Input: part model. Units: mm. Frame: model coordinates. Face numbers are marked on the shaded views. Give positions to 0.01 mm unless a question says otherwise; leave off trailing zeros. Loops run counter-clockwise (first coordinate to the right, second up) from the corner with the lowest first, then second, coordinate; pieces in that order, holes last. Notation, with made-up numbers: (66.25, 69.25) -> (97.25, 69.25) arc R26 cw to (97.25, 89.25) -> close; hole circle Ø8 at (-22.75, 75). An arc over 180 degrees is marked (long way). One line per question, with ' | ' between items.
from build123d import *

# Parameters (mm, degrees)
BOSS_EXTRUDE1_START     = -10.5
SKETCH2_R               = 3.9
BOSS_EXTRUDE1_DEPTH     = 4
BOSS_EXTRUDE2_START     = -15.5
BOSS_EXTRUDE2_OUTLINE_R = 3.9
BOSS_EXTRUDE2_DEPTH     = 5
M3_CLEARANCE_HOLE1_D    = 3.2
M3_TAPPED_HOLE1_REACH   = 32.031
M3_TAPPED_HOLE1_BORE_R  = 1.25


# Read off the part's stored shape, not the designer's step: Boss-Extrude2
with BuildPart() as part:
    # Sketch2 → Boss-Extrude1 (new body)
    with BuildSketch(Plane(origin=(0, 0, 0), x_dir=(0, 0, -1), z_dir=(1, 0, 0)).offset(BOSS_EXTRUDE1_START)):
        with BuildLine():
            Line((7.534547605, -3.521676906), (13.278030312, -2.987088741))
            ThreePointArc((13.278030312, -2.987088741), (15.983180385, -0.317229866), (13.9, 2.861817604))
            Line((13.9, 2.861817604), (3.358528015, 6.176957176))
            Line((3.358528015, 6.176957176), (-4.343824749, 12.551142838))
            ThreePointArc((-4.343824749, 12.551142838), (-7.820620852, 12.799917558), (-9.185849324, 9.592714537))
            Line((-9.185849324, 9.592714537), (-6.737511079, -1.488604871))
            ThreePointArc((-6.737511079, -1.488604871), (-6.093212803, -3.237708717), (-5.004243793, -4.750530924))
            ThreePointArc((-5.004243793, -4.750530924), (-4.613436828, -5.232032538), (-4.301751563, -5.768153965))
            ThreePointArc((-4.301751563, -5.768153965), (-3.563882529, -6.593562507), (-2.5, -6.9))
            Line((-2.5, -6.9), (2.5, -6.9))
            ThreePointArc((2.5, -6.9), (3.563882529, -6.593562507), (4.301751563, -5.768153965))
            ThreePointArc((4.301751563, -5.768153965), (5.622657157, -4.219686633), (7.534547605, -3.521676906))
        make_face()
        Circle(SKETCH2_R, mode=Mode.SUBTRACT)
    extrude(amount=BOSS_EXTRUDE1_DEPTH)

    # Boss-Extrude2 outline → Boss-Extrude2 (add)
    with BuildSketch(Plane(origin=(0, 0, 0), x_dir=(0, 0, -1), z_dir=(1, 0, 0)).offset(BOSS_EXTRUDE2_START)):
        with BuildLine():
            ThreePointArc((5.004243793, -4.750530924), (0, 6.9), (-5.004243793, -4.750530924))
            ThreePointArc((-5.004243793, -4.750530924), (-4.613436828, -5.232032538), (-4.301751563, -5.768153965))
            ThreePointArc((-4.301751563, -5.768153965), (-3.563882529, -6.593562507), (-2.5, -6.9))
            Line((-2.5, -6.9), (2.5, -6.9))
            ThreePointArc((2.5, -6.9), (3.563882529, -6.593562507), (4.301751563, -5.768153965))
            ThreePointArc((4.301751563, -5.768153965), (4.613436828, -5.232032538), (5.004243793, -4.750530924))
        make_face()
        Circle(BOSS_EXTRUDE2_OUTLINE_R, mode=Mode.SUBTRACT)
    extrude(amount=BOSS_EXTRUDE2_DEPTH)

    # M3 Clearance Hole1 (through all)
    with Locations(Plane.ZY.offset(10.5)):
        with Locations((-13, 0), (6.256496681, 10.239934047)):
            Hole(M3_CLEARANCE_HOLE1_D / 2)

    # M3 Tapped Hole1 bore → M3 Tapped Hole1 (cut, up to next)
    with BuildSketch(Plane(origin=(0, -6.9, 0), x_dir=(-1, 0, 0), z_dir=(0, -1, 0)), mode=Mode.PRIVATE) as m3_tapped_hole1_sk1:
        with Locations((11, 0)):
            Circle(M3_TAPPED_HOLE1_BORE_R)
    m3_tapped_hole1_tool1 = extrude(m3_tapped_hole1_sk1.sketch, amount=-M3_TAPPED_HOLE1_REACH, mode=Mode.PRIVATE) & part.part
    add(m3_tapped_hole1_tool1.solids().sort_by_distance((-11, -6.9, 0))[0], mode=Mode.SUBTRACT)


solid = part.part
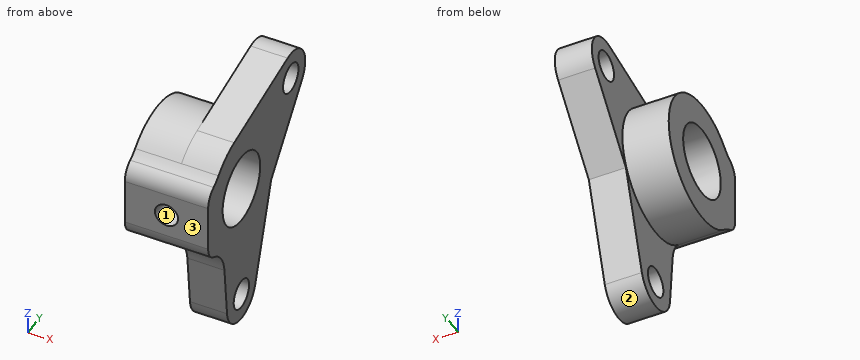
1. Pin query (flat end, axial travel): P1, Ø4, axis at x = -13.5, y = 7.5, coming from the -Z side; P2, Ø3, axis at x = -11, z = 0, coming from the +Y side. Return the tip coordinate at first contact, or that it passes through.
Determined:
P1: stops at z = -4.17 | P2: stops at y = 10.13
2. Pull-direction query (Z, two-part tool) for the marked faces 1, 2 and 3; classes: pulls with the +Z half, pulls with the -Z half, needs draft (parallel to the pull), parting line crosses it, or undercut.
Determined:
face 1: undercut | face 2: pulls with the -Z half | face 3: needs draft
3. Section query C-C (y = 3.5). Output: boundary loops of the cut face in (x, z), then the cut area to 3 significant figures.
Determined:
outline: (-15.5, -5.95) -> (-10.5, -5.95) -> (-10.5, -11.87) -> (-6.5, -11.87) -> (-6.5, -1.72) -> (-15.5, -1.72) -> close; (-15.5, 1.72) -> (-6.5, 1.72) -> (-6.5, 7.84) -> (-10.5, 7.84) -> (-10.5, 5.95) -> (-15.5, 5.95) -> close | area: 107 mm2
4. Section query A-A (x = -13.75). Output: boundary loops of the cut face in (y, z), then the cut area to 3 significant figures.
Determined:
outline: (-6.9, -2.5) arc R2 ccw to (-5.77, -4.3) arc R4 cw to (-4.75, -5) arc R6.9 ccw (long way) to (-4.75, 5) arc R4 cw to (-5.77, 4.3) arc R2 ccw to (-6.9, 2.5) -> close; hole circle Ø7.8 at (0, 0) | area: 105 mm2
5. Ray query, line 1 along Z through (x, y) = (-11, -4.75); line 2 along Y through (x, z) = (-13, 0); line 3 along Y through (x, z) = (-12, 0). Return the intervals inside material, ascending. Write a range as from..to.
Determined:
line 1: z = -5..-1.25, 1.25..5 | line 2: y = -6.9..-3.9, 3.9..6.9 | line 3: y = 3.9..6.9
6. Section query B-B (z = 6). Output: boundary loops of the cut face in (x, y), then the cut area to 3 significant figures.
Determined:
outline: (-15.5, -3.41) -> (-6.5, -3.41) -> (-6.5, 8.66) -> (-10.5, 8.66) -> (-10.5, 3.41) -> (-15.5, 3.41) -> close; (-10.5, 11.82) -> (-6.5, 11.82) -> (-6.5, 13.23) -> (-10.5, 13.23) -> close | area: 88.0 mm2
7. Section query D-D (z = 0). Output: boundary loops of the cut face in (x, y).
Determined:
outline: (-15.5, -6.9) -> (-12.25, -6.9) -> (-12.25, -3.9) -> (-15.5, -3.9) -> close; (-15.5, 3.9) -> (-6.5, 3.9) -> (-6.5, 8.96) -> (-10.5, 8.96) -> (-10.5, 6.9) -> (-15.5, 6.9) -> close; (-9.75, -6.9) -> (-6.5, -6.9) -> (-6.5, -3.9) -> (-9.75, -3.9) -> close
